```python
from build123d import *

# Parameters (mm, degrees)
SKETCH1_W           = 266.954
SKETCH1_H           = 6.35
SKETCH1_W_2         = 6.35
SKETCH1_H_2         = 12.7
BOSS_EXTRUDE1_DEPTH = 6.35


with BuildPart() as part:
    # Sketch1 → Boss-Extrude1 (new body)
    with BuildSketch(Plane.XY):
        Rectangle(SKETCH1_W, SKETCH1_H)
        with Locations((130.302, 9.525)):
            Rectangle(SKETCH1_W_2, SKETCH1_H_2)
        with Locations((130.302, -9.525)):
            Rectangle(SKETCH1_W_2, SKETCH1_H_2)
    extrude(amount=BOSS_EXTRUDE1_DEPTH)


solid = part.part
```
Geometry check sheet. Reference: the model listing, model coordinates, mm. A direction names the side the tool comes from. Round coordinates to 2 decimals unless told otherwise and drop trailing zeros. Order: outer loops, then holes, each group sorted by start corner. A loop starts at its lowest first (then second) coordinate and runs counter-clockwise, first axis right, second up. Notation, with made-up numbers: (74, 12.25) - (130, 12.25) arc R23 cw to (130, 37.25) - close; hole circle Ø6 at (33, -31). An arc over 180 degrees is marked (long way). Use a Markdown table: item, result. Add a question column.
(1) Tool access check on faces 1 (the flat face through (-5, 3.175, 3)), 2 (the flat face through (130, 15.875, 3)), 3 (the flat face through (-5, -3.175, 3)). Record the directions out of +Z, -Z, +X, -X, +Y, -Y that give a thin tool (end or side, any length) a straight path to the whole face; none if there is none.
(2) Sectioned sample at C-C, the plane y = -12. Enter the section's corners in (x, z).
(3) Material ranges on line 1 along X through (y, z) = (13.5, 5.25); line 2 along Y through (x, z) = (-76, 4.5) (3 decimals), recorded low to high. Write a range as [from, to].
(4) Sectioned sample at B-B, the plane x = -97. Enter the section's corners in (y, z) (3 decimals), and give its area (3 significant figures).
(5) Sectioned sample at A-A, the plane z = 3. Enter the section's corners in (x, y) (3 decimals).
(6) Depth check by flat-ended pin: pin 1 (3 mm diameter, centred on x = -25, z = 3.5, fed in from -Y) (3 decimals); pin 2 (3 mm diameter, centred on y = 8.5, z = 3, fed in from -X). Enter the tip coordinate at first touch or a pass-through.
Answers below:
| question | item | result |
|---|---|---|
| 1 | face 1 | +Z, -Z, -X, +Y |
| 1 | face 2 | +Z, -Z, +X, -X, +Y |
| 1 | face 3 | +Z, -Z, -X, -Y |
| 2 | outline | (127.13, 0) - (133.48, 0) - (133.48, 6.35) - (127.13, 6.35) - close |
| 3 | line 1 | [127.13, 133.48] |
| 3 | line 2 | [-3.175, 3.175] |
| 4 | outline | (-3.175, 0) - (3.175, 0) - (3.175, 6.35) - (-3.175, 6.35) - close |
| 4 | area | 40.3 mm² |
| 5 | outline | (-133.477, -3.175) - (127.127, -3.175) - (127.127, -15.875) - (133.477, -15.875) - (133.477, 15.875) - (127.127, 15.875) - (127.127, 3.175) - (-133.477, 3.175) - close |
| 6 | pin 1 | y = -3.175 |
| 6 | pin 2 | x = 127.13 |
